Can you work these out from the model? Positions are in its coordinate system, mm. Face numbers are marked on the shaded views. A direction names the side the tool comes from. Round coordinates to 2 decimals unless told otherwise and drop trailing zeros. Loops run counter-clockwise (first coordinate to the right, second up) from the corner with the lowest first, then second, coordinate; pieces in that order, holes last.
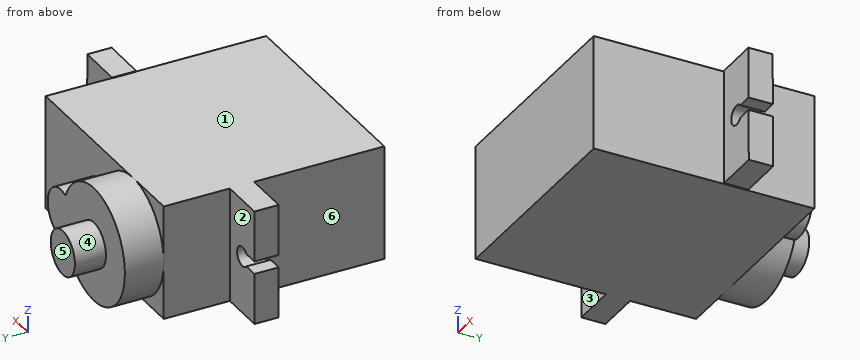
from build123d import *

# Parameters (mm, degrees)
CROQUIS1_W              = 22.5
CROQUIS1_H              = 11.8
SALIENTE_EXTRUIR1_DEPTH = 22.7
CROQUIS2_R              = 2.3
SALIENTE_EXTRUIR2_DEPTH = 4
CROQUIS3_R              = 2.3
SALIENTE_EXTRUIR3_DEPTH = 7.2
SALIENTE_EXTRUIR4_START = -6.8
SALIENTE_EXTRUIR4_DEPTH = 2.5


with BuildPart() as part:
    # Croquis1 → Saliente-Extruir1 (new body)
    with BuildSketch(Plane(origin=(0, 0, 0), x_dir=(1, 0, 0), z_dir=(0, 1, 0))):
        Rectangle(CROQUIS1_W, CROQUIS1_H)
    extrude(amount=SALIENTE_EXTRUIR1_DEPTH)

    # Croquis2 → Saliente-Extruir2 (add)
    with BuildSketch(Plane(origin=(0, 22.7, 0), x_dir=(1, 0, 0), z_dir=(0, 1, 0))):
        with BuildLine():
            ThreePointArc((0.066666667, 2.338743727), (-11.25, 0), (0.066666667, -2.338743727))
            ThreePointArc((0.066666667, -2.338743727), (3.45, 0), (0.066666667, 2.338743727))
        make_face()
        with Locations(Location((-5.35, 0, 0), (0, 0, 270))):
            Circle(CROQUIS2_R, mode=Mode.SUBTRACT)
    extrude(amount=SALIENTE_EXTRUIR2_DEPTH)

    # Croquis3 → Saliente-Extruir3 (add)
    with BuildSketch(Plane(origin=(0, 22.7, 0), x_dir=(1, 0, 0), z_dir=(0, 1, 0))):
        with Locations(Location((-5.35, 0, 0), (0, 0, 270))):
            Circle(CROQUIS3_R)
    extrude(amount=SALIENTE_EXTRUIR3_DEPTH)

    # Croquis2_3 → Saliente-Extruir4 (add)
    with BuildSketch(Plane(origin=(0, 22.7, 0), x_dir=(1, 0, 0), z_dir=(0, 1, 0)).offset(SALIENTE_EXTRUIR4_START)):
        with BuildLine():
            Line((-11.25, 5.9), (-11.25, -5.9))
            Line((-11.25, -5.9), (-15.95, -5.9))
            Line((-15.95, -5.9), (-15.95, -0.65))
            Line((-15.95, -0.65), (-14.409934208, -0.65))
            ThreePointArc((-14.409934208, -0.65), (-12.65, 0), (-14.409934208, 0.65))
            Line((-14.409934208, 0.65), (-15.95, 0.65))
            Line((-15.95, 0.65), (-15.95, 5.9))
            Line((-15.95, 5.9), (-11.25, 5.9))
        make_face()
        with BuildLine():
            Line((15.988536906, 5.794755181), (11.288638975, 5.825730005))
            Line((11.288638975, 5.825730005), (11.210872396, -5.974013736))
            Line((11.210872396, -5.974013736), (15.910770327, -6.00498856))
            Line((15.910770327, -6.00498856), (15.945369864, -0.755102574))
            Line((15.945369864, -0.755102574), (14.405337517, -0.744952943))
            ThreePointArc((14.405337517, -0.744952943), (12.649725282, -0.083368409), (14.413905022, 0.555018825))
            Line((14.413905022, 0.555018825), (15.953937369, 0.544869194))
            Line((15.953937369, 0.544869194), (15.988536906, 5.794755181))
        make_face()
    extrude(amount=-SALIENTE_EXTRUIR4_DEPTH)


solid = part.part
(1) If we section it at B-B, the plane z = -1.5: List the corners of the cut face in (x, y) for me, then the cut area to 3 significant figures.
Worked answers:
outline: (-15.95, 13.4) - (-11.25, 13.4) - (-11.25, 0) - (11.25, 0) - (11.25, 22.7) - (2.95, 22.7) - (2.95, 26.7) - (-3.61, 26.7) - (-3.61, 29.9) - (-7.09, 29.9) - (-7.09, 26.7) - (-11.06, 26.7) - (-11.06, 22.7) - (-11.25, 22.7) - (-11.25, 15.9) - (-15.95, 15.9) - close; (11.26, 13.4) - (15.96, 13.4) - (15.96, 15.9) - (11.26, 15.9) - close
area: 601 mm2
(2) For the marked faces 4, 5 and 6, which set-ups out of +Z, -Z, +X, -X, +Y, -Y let a thin tool reach every point of the face, with its end or its side?
Worked answers:
face 4: +Y
face 5: +Z, -Z, +X, -X, +Y
face 6: +Z, -Z, -X, -Y
(3) If we section it at C-C, the plane x = 0.95: List the corners of the cut face in (y, z) for me.
Worked answers:
outline: (0, -5.9) - (22.7, -5.9) - (22.7, -2.5) - (26.7, -2.5) - (26.7, 2.5) - (22.7, 2.5) - (22.7, 5.9) - (0, 5.9) - close
(4) If we section it at A-A, the plane x = -13.65: List the corners of the cut face in (y, z) for me, then the cut area to 3 significant figures.
Worked answers:
outline: (13.4, -5.9) - (15.9, -5.9) - (15.9, -1) - (13.4, -1) - close; (13.4, 1) - (15.9, 1) - (15.9, 5.9) - (13.4, 5.9) - close
area: 24.5 mm2
(5) Will these pins go through, and if not, where does the flat tip stop? P1, Ø8, axis at x = 6, y = 17.5, coming from the +Z side; P2, Ø2, axis at y = 6, z = 2.5, coming from the -X side; P3, Ø1.2, axis at x = -13.65, z = 0, coming from the -Y side; P4, Ø1, axis at x = -12.5, z = -1.5, coming from the -Y side.
Worked answers:
P1: stops at z = 5.9
P2: stops at x = -11.25
P3: passes through
P4: stops at y = 13.4
(6) If I drill on line 1 (Z direction, x = -13.65, y = 14.9); line 2 (Y direction, x = -3.5, z = 3.5); line 3 (X direction, y = 12.75, z = -1.25), over which ranges is the centre line in solid material (lowest first)?
Worked answers:
line 1: z = -5.9 to -1, 1 to 5.9
line 2: y = 0 to 26.7
line 3: x = -11.25 to 11.25
(7) If we mould it in two halves opening along Y, with no side actions, what happens to the marked faces 1, 2 and 3? For each: released by +Y, released by -Y, zero draft, split by the parting line, or undercut.
Worked answers:
face 1: zero draft
face 2: released by +Y
face 3: released by -Y
(8) If we section it at D-D, the plane z = -4.5: List the corners of the cut face in (x, y) for me.
Worked answers:
outline: (-15.95, 13.4) - (-11.25, 13.4) - (-11.25, 0) - (11.25, 0) - (11.25, 22.7) - (-1.53, 22.7) - (-1.53, 26.7) - (-9.17, 26.7) - (-9.17, 22.7) - (-11.25, 22.7) - (-11.25, 15.9) - (-15.95, 15.9) - close; (11.28, 13.4) - (15.98, 13.4) - (15.98, 15.9) - (11.28, 15.9) - close
